```python
from build123d import *

# Parameters (mm, degrees)
SKETCH1_W           = 105.585817276
SKETCH1_H           = 105.585817276
BOSS_EXTRUDE1_DEPTH = 3.175
BOSS_EXTRUDE2_DEPTH = 3.175
CUT_EXTRUDE2_DEPTH  = 90.210847709
CIRPATTERN1_COUNT   = 4
SKETCH4_R           = 8.001
CUT_EXTRUDE3_DEPTH  = 3.175
SKETCH5_W           = 44.791908638
SKETCH5_H           = 3
BOSS_EXTRUDE3_DEPTH = 2.54
CIRPATTERN2_COUNT   = 4


with BuildPart() as part:
    # Sketch1 → Boss-Extrude1 (new body)
    with BuildSketch(Plane(origin=(0, 0, 0), x_dir=(1, 0, 0), z_dir=(0, 1, 0))):
        Rectangle(SKETCH1_W, SKETCH1_H)
    extrude(amount=BOSS_EXTRUDE1_DEPTH)

    # Sketch2 → Boss-Extrude2 (add)
    with BuildSketch(Plane(origin=(0, 0, 0), x_dir=(1, 0, 0), z_dir=(0, 1, 0))):
        with BuildLine():
            Line((-52.792908638, 35.921454319), (-52.792908638, 16.871454319))
            ThreePointArc((-52.792908638, 16.871454319), (-56.083715202, 22.19609119), (-62.317908638, 21.633954319))
            ThreePointArc((-62.317908638, 21.633954319), (-68.552102074, 21.071817448), (-71.842908638, 26.396454319))
            ThreePointArc((-71.842908638, 26.396454319), (-68.552102074, 31.72109119), (-62.317908638, 31.158954319))
            ThreePointArc((-62.317908638, 31.158954319), (-56.083715202, 30.596817448), (-52.792908638, 35.921454319))
        make_face()
    boss_extrude2 = extrude(amount=BOSS_EXTRUDE2_DEPTH)

    # Sketch2<3> → Cut-Extrude2 (cut, through all)
    with BuildSketch(Plane(origin=(0, 0, 0), x_dir=(1, 0, 0), z_dir=(0, 1, 0))):
        with BuildLine():
            Line((-52.792908638, -35.921454319), (-52.792908638, -16.871454319))
            ThreePointArc((-52.792908638, -16.871454319), (-49.502102074, -22.19609119), (-43.267908638, -21.633954319))
            ThreePointArc((-43.267908638, -21.633954319), (-37.033715202, -21.071817448), (-33.742908638, -26.396454319))
            ThreePointArc((-33.742908638, -26.396454319), (-37.033715202, -31.72109119), (-43.267908638, -31.158954319))
            ThreePointArc((-43.267908638, -31.158954319), (-49.502102074, -30.596817448), (-52.792908638, -35.921454319))
        make_face()
    cut_extrude2 = extrude(amount=CUT_EXTRUDE2_DEPTH, mode=Mode.SUBTRACT)

    # CirPattern1: Boss-Extrude2, Cut-Extrude2 ×4 about axis
    cirpattern1_axis = Axis((0, 0, 0), (0, 1, 0))
    add([boss_extrude2.rotate(cirpattern1_axis, i * 360 / CIRPATTERN1_COUNT) for i in range(1, CIRPATTERN1_COUNT)])
    add([cut_extrude2.rotate(cirpattern1_axis, i * 360 / CIRPATTERN1_COUNT) for i in range(1, CIRPATTERN1_COUNT)], mode=Mode.SUBTRACT)

    # Sketch4 → Cut-Extrude3 (cut)
    with BuildSketch(Plane(origin=(0, 3.175, 0), x_dir=(1, 0, 0), z_dir=(0, 1, 0))):
        with Locations(Location((0, 0, 0), (0, 0, 270))):
            Circle(SKETCH4_R)
    extrude(amount=-CUT_EXTRUDE3_DEPTH, mode=Mode.SUBTRACT)

    # Sketch5 → Boss-Extrude3 (add)
    with BuildSketch(Plane(origin=(0, 3.175, 0), x_dir=(1, 0, 0), z_dir=(0, 1, 0))):
        with Locations((-30.396954319, -1.5)):
            Rectangle(SKETCH5_W, SKETCH5_H)
        with Locations((-30.396954319, 1.5)):
            Rectangle(SKETCH5_W, SKETCH5_H)
    boss_extrude3 = extrude(amount=BOSS_EXTRUDE3_DEPTH)

    # CirPattern2: Boss-Extrude3 ×4 about axis
    cirpattern2_axis = Axis((0, 0, 0), (0, 1, 0))
    for i in range(1, CIRPATTERN2_COUNT):
        add(boss_extrude3.rotate(cirpattern2_axis, i * 360 / CIRPATTERN2_COUNT))


solid = part.part
```
Here's how the part is built. I have some questions about the finished solid (model axes, mm). A direction names the side the tool comes from. Coordinates: 2 decimals unless noted, no trailing zeros. Order: outer loops, then holes, each group sorted by start corner. A loop starts at its lowest first (then second) coordinate and runs counter-clockwise, first axis right, second up.
Item 1: Which directions (+Z, -Z, +X, -X, +Y, -Y) give clear straight access to the entire face, cutting with the end or side of a thin tool? Please do faces 1 (the face through (52.793, 2, 0)), 2 (the face through (-52.793, 2, 44)), 3 (the face through (0, 2, -52.793)), 4 (the face through (44, 2, 52.793)).
Response values:
face 1: -Z, +X, +Y, -Y
face 2: +Z, -X, +Y, -Y
face 3: -Z, -X, +Y, -Y
face 4: +Z, +X, +Y, -Y
Item 2: If we section it at B-B, the plane x = 12: List the corners of the cut face in (y, z) for me (3 decimals), then the cut area to 3 significant figures.
Response values:
outline: (0, -52.793) - (3.175, -52.793) - (3.175, -3) - (5.715, -3) - (5.715, 3) - (3.175, 3) - (3.175, 52.793) - (0, 52.793) - close
area: 350 mm2
Item 3: I need wall thicknesses on probe 1 along X at (y, z) = (1.5, 0.5); probe 2 along X at (y, z) = (1.8, 47); probe 3 along X at (y, z) = (4.45, 30). Which ranges of each line are inside material? Lowest first, please.
Response values:
probe 1: x = -52.79 to -7.99, 7.99 to 52.79
probe 2: x = -52.79 to 22.82, 29.97 to 52.79
probe 3: x = -3 to 3
Item 4: If we section it at A-A, the plane y = 4.65: List the corners of the cut face in (x, z) for me, then the cut area to 3 significant figures.
Response values:
outline: (-52.79, -3) - (-8, -3) - (-8, 3) - (-52.79, 3) - close; (-3, -52.79) - (3, -52.79) - (3, -8) - (-3, -8) - close; (-3, 8) - (3, 8) - (3, 52.79) - (-3, 52.79) - close; (8, -3) - (52.79, -3) - (52.79, 3) - (8, 3) - close
area: 1,080 mm2
Item 5: I'm going to push flat-ended pins straight in: pin 1 Ø1.3 at (x, y) = (23.5, 4.5) entering from +Z; pin 2 Ø1.5 at (x, z) = (12.5, 38) entering from +Y (3 decimals); pin 3 Ø1.3 at (x, y) = (-40.5, 4) entering from -Z. Where does each tip first touch, or does it pass through?
Response values:
pin 1: stops at z = 3
pin 2: stops at y = 3.175
pin 3: stops at z = -3
Item 6: Thinking about a two-plate mould opening in Z: for faces 5 (the face through (-52.793, 2, 0)), 6 (the face through (2.403, 1.61, 7.632)), 7 (the face through (44, 2, -52.793)), which applies, pulls with the +Z half, pulls with the -Z half, needs draft (parallel to the pull), parting line crosses it, or undercut?
Response values:
face 5: needs draft
face 6: undercut
face 7: pulls with the -Z half
Item 7: If we section it at D-D, the plane z = 24.5: List the corners of the cut face in (x, y) for me (3 decimals).
Response values:
outline: (-34.053, 0) - (71.533, 0) - (71.533, 3.175) - (3, 3.175) - (3, 5.715) - (-3, 5.715) - (-3, 3.175) - (-34.053, 3.175) - close
Item 8: If we section it at C-C, the plane z = 49: List the corners of the cut face in (x, y) for me (3 decimals), then the cut area to 3 significant figures.
Response values:
outline: (-52.793, 0) - (22.419, 0) - (22.419, 3.175) - (3, 3.175) - (3, 5.715) - (-3, 5.715) - (-3, 3.175) - (-52.793, 3.175) - close; (30.374, 0) - (52.793, 0) - (52.793, 3.175) - (30.374, 3.175) - close
area: 325 mm2
